```python
from build123d import *

# Parameters (mm, degrees)
F0_R      = 2.5
F1_DEPTH  = 2
F2_W      = 9
F2_H      = 6.5
F3_DEPTH  = 1
F4_W      = 3.5
F4_H      = 5
F5_DEPTH  = 3.5
F6_R      = 0.5
F7_DEPTH  = 25
F8_R      = 2
F9_W      = 1
F9_H      = 1.5
F10_DEPTH = 1
F11_W     = 1
F11_H     = 1.5
F12_DEPTH = 1
F13_R     = 1
F15_W     = 0.5
F15_H     = 1.5
F14_W     = 0.5
F14_H     = 1.5
F16_DEPTH = 25


with BuildPart() as f1:
    # F0 (on Front) → F1 (new body)
    with BuildSketch(Plane.XZ):
        Circle(F0_R)
    extrude(amount=F1_DEPTH)

    # F2 (on Front) → F3 (join)
    with BuildSketch(Plane.XZ):
        Rectangle(F2_W, F2_H)
    extrude(amount=-F3_DEPTH)

    # F4 (on face) → F5 (join)
    with BuildSketch(Plane(origin=(0, 1, 0), x_dir=(-1, 0, 0), z_dir=(0, 1, 0))):
        Rectangle(F4_W, F4_H)
    extrude(amount=F5_DEPTH)

    # F6 (on face) → F7 (cut)
    with BuildSketch(Plane(origin=(-1.75, 0, 0), x_dir=(0, -1, 0), z_dir=(-1, 0, 0))):
        with Locations((-3.5, 0)):
            Circle(F6_R)
    extrude(amount=-F7_DEPTH, mode=Mode.SUBTRACT)

    # F8
    f8_edges = [f1.edges().sort_by_distance(p)[0] for p in [
        (0, 4.5, -2.5),
        (0, 4.5, 2.5),
    ]]
    fillet(f8_edges, radius=F8_R)

    # F9 (on face) → F10 (cut)
    with BuildSketch(Plane(origin=(-4.5, 0, 0), x_dir=(0, -1, 0), z_dir=(-1, 0, 0))):
        with Locations((-0.5, 0)):
            Rectangle(F9_W, F9_H)
    extrude(amount=-F10_DEPTH, mode=Mode.SUBTRACT)

    # F11 (on face) → F12 (cut)
    with BuildSketch(Plane.YZ.offset(4.5)):
        with Locations((0.5, 0)):
            Rectangle(F11_W, F11_H)
    extrude(amount=-F12_DEPTH, mode=Mode.SUBTRACT)

    # F13
    f13_edges = [f1.edges().sort_by_distance(p)[0] for p in [
        (4.5, 0.5, 3.25),
        (4.5, 0.5, -3.25),
        (-4.5, 0.5, -3.25),
        (-4.5, 0.5, 3.25),
    ]]
    fillet(f13_edges, radius=F13_R)

    # F15 (on face) + F14 (on face) → F16 (cut)
    with BuildSketch(Plane(origin=(0, 1, 0), x_dir=(-1, 0, 0), z_dir=(0, 1, 0))):
        with Locations((3.25, 0)):
            Rectangle(F15_W, F15_H)
    with BuildSketch(Plane(origin=(0, 1, 0), x_dir=(-1, 0, 0), z_dir=(0, 1, 0))):
        with Locations((-3.25, 0)):
            Rectangle(F14_W, F14_H)
    extrude(amount=-F16_DEPTH, mode=Mode.SUBTRACT)


solid = f1.part
```
The listing builds one solid part. Answer for the finished solid, in the listing's coordinates (mm). A direction names the side the tool comes from. Coordinates: 2 decimals unless noted, no trailing zeros. Loops run counter-clockwise (first coordinate to the right, second up) from the corner with the lowest first, then second, coordinate; pieces in that order, holes last. Notation, with made-up numbers: M 44.5,10 L 77.5,10 A26 cw 77.5,38 Z; hole C 80.5,86 d11. An arc over 180 degrees is marked long. Answer as CSV lines item,"result". Start each with the question number.
(1) The mould has two halves that part along Z. Classify faces 5 (the cylindrical face through (4.215, 0.507, -2.949)), 6 (the flat face through (3.8, 0.5, 0.75)), 7 (the flat face through (4.5, 0.5, -1.5)): pulls with the +Z half, pulls with the -Z half, needs draft (parallel to the pull), parting line crosses it, or undercut.
(2) Find the intervals of material crossed by L1, parallel to X at y = 4.25, z = -1; L2, parallel to Y at x = -3.25, z = 1; L3, parallel to Z at x = 0.45, y = 3.5, in increasing order. Write a range as [from, to].
(3) The part is cut by section D-D (z = 1.75). Give the vertices of the cut face in (x, y).
(4) The part is cut by section A-A (x = 0). Give the vertices of the cut face in (y, z), and give its area (3 significant figures).
(5) The part is cut by section B-B (z = 0). Give the vertices of the cut face in (x, y), and give its area (4 significant figures).
(6) The part is cut by section C-C (y = 3.5). Give the vertices of the cut face in (x, z), and give its area (3 significant figures).
(7) Given pin 1 (1 mm diameter, centred on y = 3, z = -0.5, fed in from +X); pin 2 (1.1 mm diameter, centred on y = 0.5, z = 0, fed in from +X); pin 3 (0.5 mm diameter, centred on x = -1, y = 1.5, fed in from -Z), each flat-ended and moving along its own axis, determine where each tip first touches the part or whether it passes through.
(8) For faces 1 (the flat face through (-3, 0.5, 0)), 2 (the flat face through (-1.75, 2.7, 0)), 3 (the flat face through (1.75, 2.7, 0)), 4 (the flat face through (0, 2, 2.5)), determine the directions among +Z, -Z, +X, -X, +Y, -Y from which every point of the face is accessible in a straight line to the end or side of a thin tool.
Determined:
1,face 5,"pulls with the -Z half"
1,face 6,"undercut"
1,face 7,"needs draft"
2,L1,"[-1.75, 1.75]"
2,L2,"[0, 1]"
2,L3,"[-2.23, -0.5], [0.5, 2.23]"
3,outline,"M -4.5,0 L -1.79,0 L -1.79,-2 L 1.79,-2 L 1.79,0 L 4.5,0 L 4.5,1 L 1.75,1 L 1.75,4.06 L -1.75,4.06 L -1.75,1 L -4.5,1 Z"
4,outline,"M -2,-2.5 L 0,-2.5 L 0,-3.25 L 1,-3.25 L 1,-2.5 L 2.5,-2.5 A2 ccw 4.5,-0.5 L 4.5,0.5 A2 ccw 2.5,2.5 L 1,2.5 L 1,3.25 L 0,3.25 L 0,2.5 L -2,2.5 Z; hole C 3.5,0 d1"
4,area,"31.5 mm2"
5,outline,"M -3,0 L -2.5,0 L -2.5,-2 L 2.5,-2 L 2.5,0 L 3,0 L 3,1 L 1.75,1 L 1.75,3 L -1.75,3 L -1.75,1 L -3,1 Z; M -1.75,4 L 1.75,4 L 1.75,4.5 L -1.75,4.5 Z"
5,area,"24.75 mm2"
6,outline,"M -1.75,-2.23 L 1.75,-2.23 L 1.75,-0.5 L -1.75,-0.5 Z; M -1.75,0.5 L 1.75,0.5 L 1.75,2.23 L -1.75,2.23 Z"
6,area,"12.1 mm2"
7,pin 1,"x = 1.75"
7,pin 2,"x = 3"
7,pin 3,"z = -2.5"
8,face 1,"-X, +Y, -Y"
8,face 2,"+Z, -Z, -X, +Y"
8,face 3,"+Z, -Z, +X, +Y"
8,face 4,"+Z, +X, -X, +Y"
